```python
from build123d import *

# Parameters (mm, degrees)
F0_W      = 25.4
F0_H      = 25.4
F1_DEPTH  = 25.4
F3_D      = 4.7752
F3_DEPTH  = 3.81
F3_TIP    = 1.434614814
F6_D      = 4.7752
F6_DEPTH  = 3.81
F6_TIP    = 1.434614814
F11_D     = 4.7752
F11_DEPTH = 3.81
F11_TIP   = 1.434614814
F14_D     = 4.7752
F14_DEPTH = 3.81
F14_TIP   = 1.434614814
F15_D     = 4.7752
F15_DEPTH = 3.81
F15_TIP   = 1.434614814
F18_D     = 4.7752
F18_DEPTH = 3.81
F18_TIP   = 1.434614814


with BuildPart() as f1:
    # F0 (on Top) → F1 (new body)
    with BuildSketch(Plane.XY):
        with Locations((12.7, 12.7)):
            Rectangle(F0_W, F0_H)
    extrude(amount=F1_DEPTH)

    # F3
    with Locations(Plane.XY.offset(25.4)):
        with Locations((11.7311347276, 13.4724741802)):
            Hole(F3_D / 2, depth=F3_DEPTH)
            with Locations((0, 0, -(F3_DEPTH + F3_TIP / 2))):  # 118° drill point
                Cone(0, F3_D / 2, F3_TIP, mode=Mode.SUBTRACT)

    # F6
    with Locations(Plane(origin=(0, 0, 0), x_dir=(1, 0, 0), z_dir=(0, 0, -1))):
        with Locations((7.5152567588, -6.1405156739), (17.7800003439, -6.1405156739), (7.5152567588, -12.3726800084), (17.7800003439, -12.3726800084), (17.7800003439, -18.7881439924), (7.5152567588, -18.7881439924)):
            Hole(F6_D / 2, depth=F6_DEPTH)
            with Locations((0, 0, -(F6_DEPTH + F6_TIP / 2))):  # 118° drill point
                Cone(0, F6_D / 2, F6_TIP, mode=Mode.SUBTRACT)

    # F11
    with Locations(Plane(origin=(0, 0, 0), x_dir=(0, -1, 0), z_dir=(-1, 0, 0))):
        with Locations((-17.9789844365, 18.0393166689), (-6.9078497357, 6.9310304664)):
            Hole(F11_D / 2, depth=F11_DEPTH)
            with Locations((0, 0, -(F11_DEPTH + F11_TIP / 2))):  # 118° drill point
                Cone(0, F11_D / 2, F11_TIP, mode=Mode.SUBTRACT)

    # F14
    with Locations(Plane(origin=(0, 25.4, 0), x_dir=(-1, 0, 0), z_dir=(0, 1, 0))):
        with Locations((-4.7665690069, 20.8159134085), (-12.8613589332, 12.7752926201), (-20.2033963729, 5.4823870097)):
            Hole(F14_D / 2, depth=F14_DEPTH)
            with Locations((0, 0, -(F14_DEPTH + F14_TIP / 2))):  # 118° drill point
                Cone(0, F14_D / 2, F14_TIP, mode=Mode.SUBTRACT)

    # F15
    with Locations(Plane.YZ.offset(25.4)):
        with Locations((4.6540303156, 19.0304033458), (4.6540303156, 6.6524622962), (11.0050151125, 12.8738358617), (17.4208078533, 19.0304033458), (17.4856130034, 6.6524622962)):
            Hole(F15_D / 2, depth=F15_DEPTH)
            with Locations((0, 0, -(F15_DEPTH + F15_TIP / 2))):  # 118° drill point
                Cone(0, F15_D / 2, F15_TIP, mode=Mode.SUBTRACT)

    # F18
    with Locations(Plane.XZ):
        with Locations((7.725846488, 19.1752817482), (17.8987849504, 19.1752817482), (17.8987849504, 6.6132424399), (7.725846488, 6.6132424399)):
            Hole(F18_D / 2, depth=F18_DEPTH)
            with Locations((0, 0, -(F18_DEPTH + F18_TIP / 2))):  # 118° drill point
                Cone(0, F18_D / 2, F18_TIP, mode=Mode.SUBTRACT)


solid = f1.part
```
Read the model definition and answer for the solid it produces. Units are mm, in the model's axes. A direction names the side the tool comes from. Give positions to 0.01 mm unless a question says otherwise; leave off trailing zeros. Write item = value, one per line. Start each with the question number.
Item 1: A tool of negligible diameter and unlimited length cuts with its end or side. For faces 5 (the cylindrical face through (19.659, 1.932, 8.227)), 6 (the cylindrical face through (23.47, 5.17, 4.32)), 7 (the cylindrical face through (9.454, 14.19, 23.468)), 8 (the cylindrical face through (5.31, 7.055, 1.932)), 9 (the flat face through (13, 25.4, 10)), from which of +Z, -Z, +X, -X, +Y, -Y can it reach the whole face along a straight path? Write none if from no direction.
Item 2: Each of these flat-tipped pins is pushed along its axis until it touches: P1, Ø4.5, axis at y = 11.01, z = 12.87, coming from the +X side; P2, Ø4, axis at x = 12.86, z = 12.78, coming from the +Y side; P3, Ø4.5, axis at x = 4.77, z = 20.82, coming from the +Y side. Where does it stop, or does it pass through?
Item 3: The mould has two halves that part along X. Classify faces 1 (the conical face through (7.397, 4.995, 18.923)), 2 (the cylindrical face through (14.14, 23.47, 14.79)), 3 (the conical face through (20.405, 4.6, 19.442)), 4 (the cylindrical face through (23.47, 12.9, 11.42)): +X half, -X half, draft (parallel to the pull), parting line (faces both ways), or undercut.
Item 4: Find the intervals of material crossed by probe 1 along X at (y, z) = (1.25, 19); probe 2 along Y at (x, z) = (7.5, 2.25); probe 3 along Z at (x, y) = (23, 18), in increasing order. Write a range as [from, to].
Response:
q1.face_5 = -Y
q1.face_6 = +X
q1.face_7 = +Z
q1.face_8 = -Z
q1.face_9 = +Z, -Z, +X, -X, +Y
q2.P1 = 21.51
q2.P2 = 21.36
q2.P3 = 21.51
q3.face_1 = undercut
q3.face_2 = undercut
q3.face_3 = +X half
q3.face_4 = draft
q4.probe_1 = [0, 5.34], [10.11, 15.52], [20.28, 25.4]
q4.probe_2 = [0, 3.75], [8.53, 9.99], [14.76, 16.4], [21.18, 25.4]
q4.probe_3 = [0, 4.32], [8.98, 16.71], [21.35, 25.4]
